Can you work these out from the model? Positions are in its coordinate system, mm. A direction names the side the tool comes from. Coordinates: 2 decimals unless noted, no trailing zeros. Loops run counter-clockwise (first coordinate to the right, second up) from the corner with the lowest first, then second, coordinate; pieces in that order, holes last.
```python
from build123d import *

# Parameters (mm, degrees)
SKETCH1_R           = 2.5
BOSS_EXTRUDE1_DEPTH = 3
SKETCH2_W           = 42
SKETCH2_H           = 45
BOSS_EXTRUDE2_DEPTH = 3
SKETCH3_R           = 12.5
SKETCH3_R_2         = 1.5
CUT_EXTRUDE1_DEPTH  = 13


with BuildPart() as part:
    # Sketch1 → Boss-Extrude1 (new body)
    with BuildSketch(Plane.XY):
        Polygon((40, 0), (0, 0), (0, -100), (82, -100), (82, -66), (40, -66), align=None)
        with Locations((30, -5)):
            Circle(SKETCH1_R, mode=Mode.SUBTRACT)
        with Locations((10, -5)):
            Circle(SKETCH1_R, mode=Mode.SUBTRACT)
        with Locations((10, -27.5)):
            Circle(SKETCH1_R, mode=Mode.SUBTRACT)
        with Locations((10, -50)):
            Circle(SKETCH1_R, mode=Mode.SUBTRACT)
        with Locations((10, -72.5)):
            Circle(SKETCH1_R, mode=Mode.SUBTRACT)
        with Locations((10, -95)):
            Circle(SKETCH1_R, mode=Mode.SUBTRACT)
        with Locations((30, -27.5)):
            Circle(SKETCH1_R, mode=Mode.SUBTRACT)
        with Locations((30, -50)):
            Circle(SKETCH1_R, mode=Mode.SUBTRACT)
        with Locations((30, -72.5)):
            Circle(SKETCH1_R, mode=Mode.SUBTRACT)
        with Locations((30, -95)):
            Circle(SKETCH1_R, mode=Mode.SUBTRACT)
    extrude(amount=BOSS_EXTRUDE1_DEPTH)

    # Sketch2 → Boss-Extrude2 (add)
    with BuildSketch(Plane(origin=(0, -66, 0), x_dir=(1, 0, 0), z_dir=(0, 1, 0))):
        with Locations((61, -22.5)):
            Rectangle(SKETCH2_W, SKETCH2_H)
    extrude(amount=BOSS_EXTRUDE2_DEPTH)

    # Sketch3 → Cut-Extrude1 (cut)
    with BuildSketch(Plane.XZ.offset(66)):
        with Locations((61, 24)):
            Circle(SKETCH3_R)
        with Locations((45.5, 39.5)):
            Circle(SKETCH3_R_2)
        with Locations((45.5, 8.5)):
            Circle(SKETCH3_R_2)
        with Locations((76.5, 8.5)):
            Circle(SKETCH3_R_2)
        with Locations((76.5, 39.5)):
            Circle(SKETCH3_R_2)
    extrude(amount=-CUT_EXTRUDE1_DEPTH, mode=Mode.SUBTRACT)


solid = part.part
```
(1) If I drill on probe 1 along Y at (x, z) = (30, 1.9); probe 2 along Z at (x, y) = (22, -52.5); probe 3 along Y at (x, z) = (63, 4.5), over which ranges is the centre line in solid material (lowest first)?
Check values:
probe 1: y = -100 to -97.5, -92.5 to -75, -70 to -52.5, -47.5 to -30, -25 to -7.5, -2.5 to 0
probe 2: z = 0 to 3
probe 3: y = -66 to -63
(2) I want a section at A-A on y = -27.5. Write out the boundary of the cut face in (x, z).
Check values:
outline: (0, 0) - (7.5, 0) - (7.5, 3) - (0, 3) - close; (12.5, 0) - (27.5, 0) - (27.5, 3) - (12.5, 3) - close; (32.5, 0) - (40, 0) - (40, 3) - (32.5, 3) - close
(3) I want a section at D-D on z = 24. Write out the boundary of the cut face in (x, y), then the cut area to 3 significant figures.
Check values:
outline: (40, -66) - (48.5, -66) - (48.5, -63) - (40, -63) - close; (73.5, -66) - (82, -66) - (82, -63) - (73.5, -63) - close
area: 51.0 mm2
(4) Which directions (+Z, -Z, +X, -X, +Y, -Y) give clear straight access to the entire face, cutting with the end or side of a thin tool? Please do faces 4 (the flat face through (40, -65, 24)), 5 (the flat face through (56, -63, 12)), 6 (the cylindrical face through (44.3, -64.5, 38.6)).
Check values:
face 4: +Z, -X, +Y, -Y
face 5: +Z, -Z, +X, +Y
face 6: +Y, -Y
(5) I want a section at C-C on x = 30. Write out the boundary of the cut face in (y, z), then the cut area to 3 significant figures.
Check values:
outline: (-100, 0) - (-97.5, 0) - (-97.5, 3) - (-100, 3) - close; (-92.5, 0) - (-75, 0) - (-75, 3) - (-92.5, 3) - close; (-70, 0) - (-52.5, 0) - (-52.5, 3) - (-70, 3) - close; (-47.5, 0) - (-30, 0) - (-30, 3) - (-47.5, 3) - close; (-25, 0) - (-7.5, 0) - (-7.5, 3) - (-25, 3) - close; (-2.5, 0) - (0, 0) - (0, 3) - (-2.5, 3) - close
area: 225 mm2
(6) I want a section at B-B on x = 61. Write out the boundary of the cut face in (y, z).
Check values:
outline: (-100, 0) - (-63, 0) - (-63, 11.5) - (-66, 11.5) - (-66, 3) - (-100, 3) - close; (-66, 36.5) - (-63, 36.5) - (-63, 45) - (-66, 45) - close
(7) If we mould it in two halves opening along X, with no side actions, what happens to faces 1 (the flat face through (31, -60, 3)), 2 (the flat face through (40, -32, 1)), 3 (the cylindrical face through (9.67, -2.52, 1.48))? For each: released by +X, released by -X, zero draft, split by the parting line, or undercut.
Check values:
face 1: zero draft
face 2: released by +X
face 3: undercut
(8) I'm going to push flat-ended pins straight in: pin 1 (3.5 mm diameter, centred on x = 45.5, z = 8.5, fed in from -Y); pin 2 (2.5 mm diameter, centred on x = 76.5, z = 39.5, fed in from -Y); pin 3 (8 mm diameter, centred on x = 30, y = -95, fed in from -Z); pin 4 (5 mm diameter, centred on x = 29.5, y = -87.5, fed in from +Z). Where does each tip first touch, or does it pass through?
Check values:
pin 1: stops at y = -66
pin 2: passes through
pin 3: stops at z = 0
pin 4: stops at z = 3
